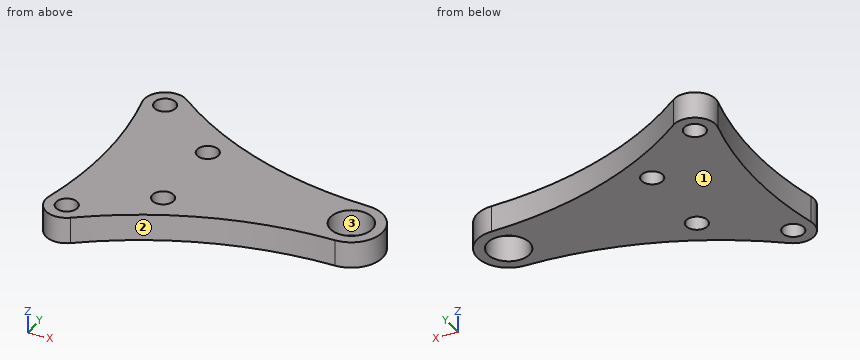
Autodesk Inventor part; units mm, degrees
ref_plane "XY Plane" through (0, 0, 0) normal (0, 0, 1) x (1, 0, 0)
sketch "Sketch1" plane through (0, 0, 0) normal (0, 0, 1) x (1, 0, 0)
  line L0 (-20, 150) -> (20, 150) construction
  line L1 (20, 150) -> (20, -150) construction
  line L2 (20, -150) -> (-20, -150) construction
  line L3 (-20, -150) -> (-20, 150) construction
  circle A0 centre (-28.08, 22) radius 10.72 construction
  circle A1 centre (-28.08, -22) radius 10.72 construction
  circle A2 centre (28.08, 0) radius 10.72 construction
  line L4 (38.8, 14.9853) -> (38.8, -13.1126) construction
  circle A3 centre (28.08, 0) radius 7.5
  circle A4 centre (-28.08, 22) radius 5
  circle A5 centre (-28.08, -22) radius 5
  arc A6 (-32.9441, -20.8421) -> (-32.9441, 20.8421) centre (-120.4975, 0) ccw
  arc A7 (-25.0444, 25.9731) -> (28.1966, 7.4991) centre (29.5961, 97.4882) ccw
  arc A8 (28.1966, -7.4991) -> (-25.0444, -25.9731) centre (29.5961, -97.4882) ccw
  line L5 (-30.4975, 3.8118) -> (-30.4975, -3.8118) construction
  line L6 (0, 150) -> (0, -150) construction
  line L7 (-62, -108) -> (-20, -108) construction
  line L8 (-20, -108) -> (-20, -150) construction
  line L9 (-20, -150) -> (-62, -150) construction
  line L10 (-62, -150) -> (-62, -108) construction
  line L11 (-62, 150) -> (-20, 150) construction
  line L12 (-20, 150) -> (-20, 108) construction
  line L13 (-20, 108) -> (-62, 108) construction
  line L14 (-62, 108) -> (-62, 150) construction
  circle A9 centre (-41, -129) radius 6 construction
  line L15 (-70.4975, 7.5) -> (-30.4975, 7.5)
  line L16 (-30.4975, 7.5) -> (-30.4975, -7.5)
  line L17 (-30.4975, -7.5) -> (-70.4975, -7.5)
  line L18 (-70.4975, -7.5) -> (-70.4975, 7.5)
  point P0 (0, 0)
  point P1 (20, 0)
  point P2 (-29.8, 0)
  point P3 (-20, 0)
  point P4 (-62, -129)
  point P5 (-41, -108)
  point P6 (-30.4975, 0)
  point P7 (-62.9975, 0)
  point P8 (-37.9975, 0)
  point P9 (-70.4975, 0)
  point P10 (-30.8106, -7.5)
  point P11 (-30.8106, 7.5)
  point P12 (-11.5, 10)
  point P13 (-11.5, -10)
  dimension "d0" = 40
  dimension "d1" = 300
  dimension "d2" = 21.44
  dimension "d3" = 22
  dimension "d4" = 22
  dimension "d5" = 58.8
  dimension "d6" = 28.08
  dimension "d7" = 28.08
  dimension "d9" = 90
  dimension "d12" = 15
  dimension "d38" = 10
  dimension "d40" = 42
  dimension "d41" = 12
  dimension "d42" = 15
  dimension "d43" = 40
  dimension "d44" = 25
  dimension "d45" = 7.5
  dimension "d46" = 7.5
  dimension "d48" = 90
  dimension "d49" = 16.58
  dimension "d50" = 12
  dimension "d51" = 10
extrude "Extrusion1" add sketch "Sketch1" against normal blind 6.35 contours A3 | A3 A8 A5 A6 L17 L16 L15 A4 A7 | A4 | A5 | L15 L16 A6 | A6 L16 L17
hole "Hole1" at (-28.08, 22, 0) at (-28.08, -22, 0) direction (0, 0, -1) diameter 5.1 end through all
hole "Hole3" at (28.08, 0, 0) direction (0, 0, -1) diameter 10 end through all
ref_plane "Work Plane2" through (-30.4975, 0, 0) normal (1, 0, 0) x (0, 1, 0)
ref_plane "Work Plane3" through (0, 150, 0) normal (-1, 0, 0) x (0, -1, 0)
hole "Hole4" at (-62.9975, 0, 0) at (-37.9975, 0, 0) at (-11.5, 10, 0) at (-11.5, -10, 0) direction (0, 0, -1) diameter 5.1 end through all
properties part number "XZ Plate2"
Geometry check sheet. Reference: the model listing, model coordinates, mm. Face numbers are marked on the shaded views. Give positions to 0.01 mm unless a question says otherwise; leave off trailing zeros. Order: outer loops, then holes, each group sorted by start corner. A loop starts at its lowest first (then second) coordinate and runs counter-clockwise, first axis right, second up.
1. Section check C-C, the plane z = -2. Enter the section's corners in (x, y).
2. Thickness scan on L1, parallel to X at y = 0, z = -2.25; L2, parallel to Y at x = -26, z = -6; L3, parallel to Y at x = -11.5, z = -3.75. Record the ranges inside material, lowest first.
3. Section check D-D, the plane x = 29. Enter the section's corners in (y, z).
4. Gauge pin test, flat ends, axial feed: pin 1 Ø4.5 at (x, y) = (-11.5, 10) entering from -Z; pin 2 Ø3 at (x, z) = (7.5, -2) entering from +Y; pin 3 Ø6 at (x, y) = (-11.5, -10) entering from +Z; pin 4 Ø2 at (x, z) = (20.5, -1.5) entering from +Y. Record the tip position at first contact, or that the pin passes through.
5. Section check B-B, the plane x = -11.5. Enter the section's corners in (y, z), and give its area (3 significant figures).
6. Release check for a two-part mould opening along Y. For the marked faces 1, 2 and 3 record: pulls with the +Y half, pulls with the -Y half, needs draft (parallel to the pull), parting line crosses it, or undercut.
7. Section check A-A, the plane y = 11.5. Enter the section's corners in (x, z) (3 decimals).
Values follow:
1. outline: (-32.94, -20.84) arc R5 ccw to (-25.04, -25.97) arc R90 cw to (28.2, -7.5) arc R7.5 ccw to (28.2, 7.5) arc R90 cw to (-25.04, 25.97) arc R5 ccw to (-32.94, 20.84) arc R90 cw to start; hole circle Ø5.1 at (-28.08, -22); hole circle Ø5.1 at (-28.08, 22); hole circle Ø5.1 at (-11.5, -10); hole circle Ø5.1 at (-11.5, 10); hole circle Ø10 at (28.08, 0)
2. L1: x = -30.5 to 23.08, 33.08 to 35.58
2. L2: y = -26.55 to -23.48, -20.52 to 20.52, 23.48 to 26.55
2. L3: y = -17.42 to -12.55, -7.45 to 7.45, 12.55 to 17.42
3. outline: (-7.44, -6.35) - (-4.91, -6.35) - (-4.91, 0) - (-7.44, 0) - close; (4.91, -6.35) - (7.44, -6.35) - (7.44, 0) - (4.91, 0) - close
4. pin 1: passes through
4. pin 2: stops at y = 10.64
4. pin 3: stops at z = 0
4. pin 4: stops at y = 8.06
5. outline: (-17.42, -6.35) - (-12.55, -6.35) - (-12.55, 0) - (-17.42, 0) - close; (-7.45, -6.35) - (7.45, -6.35) - (7.45, 0) - (-7.45, 0) - close; (12.55, -6.35) - (17.42, -6.35) - (17.42, 0) - (12.55, 0) - close
5. area: 156 mm2
6. face 1: needs draft
6. face 2: pulls with the -Y half
6. face 3: undercut
7. outline: (-31.235, -6.35) - (-13.562, -6.35) - (-13.562, 0) - (-31.235, 0) - close; (-9.438, -6.35) - (3.025, -6.35) - (3.025, 0) - (-9.438, 0) - close
